```python
from build123d import *

# Parameters (mm, degrees)
SKETCH_1_W      = 48
SKETCH_1_H      = 48
EXTRUDE_1_DEPTH = 60


with BuildPart() as part:
    # 草图1 → 凸台-拉伸1 (new body)
    with BuildSketch(Plane(origin=(0, 0, 0), x_dir=(1, 0, 0), z_dir=(0, 1, 0))):
        Rectangle(SKETCH_1_W, SKETCH_1_H)
    extrude(amount=EXTRUDE_1_DEPTH)

    # Surface Cut 1
    split(bisect_by=Plane(origin=(-14.481029553, 8.36062631, -7.699699993), x_dir=(0.3622245100921348, -0.20913041840877658, -0.9083269633698446), z_dir=(0.7866342252206607, -0.45416348168492593, 0.41826083681754983)), keep=Keep.TOP)


solid = part.part
```
The listing builds one solid part. Answer for the finished solid, in the listing's coordinates (mm). Coordinates: 2 decimals unless noted, no trailing zeros. Loops run counter-clockwise (first coordinate to the right, second up) from the corner with the lowest first, then second, coordinate; pieces in that order, holes last. Notation, with made-up numbers: (41.5, -30.75) - (76.5, -30.75) arc R20 ccw to (76.5, -19.75) - close; hole circle Ø8 at (19.5, 33). An arc over 180 degrees is marked (long way). Use a Markdown table: item, result. Add a question column.
1) The part is cut by section D-D, the plane z = -3. Give the vertices of the cut face in (x, y).
2) The part is cut by section B-B, the plane x = 11.5. Give the vertices of the cut face in (y, z), and give its area (3 significant figures).
3) The part is cut by section C-C, the plane y = 27. Give the vertices of the cut face in (x, z), and give its area (3 significant figures).
4) Find the intervals of material crossed by line 1 (Y direction, x = -6.5, z = 18); line 2 (X direction, y = 49.5, z = 1.5); line 3 (Z direction, x = 6, y = 48.5), in increasing order.
5) The part is cut by section A-A, the plane z = 3. Give the vertices of the cut face in (x, y).
6) Given pin 1 (12 mm diameter, centred on y = 52, z = 9.5, fed in from -X); pin 2 (12 mm diameter, centred on y = 36, z = -7.5, fed in from -X); pin 3 (6 mm diameter, centred on x = -8, z = -17.5, fed in from +Y), each flat-ended and moving along its own axis, determine where each tip first touches the part or whether it passes through.
Here are the results:
| question | item | result |
|---|---|---|
| 1 | outline | (-21.81, 0) - (24, 0) - (24, 60) - (12.83, 60) - close |
| 2 | outline | (0, -24) - (38.35, -24) - (60, -0.49) - (60, 24) - (0, 24) - close |
| 2 | area | 2,630 mm^2 |
| 3 | outline | (-20.57, 24) - (4.95, -24) - (24, -24) - (24, 24) - close |
| 3 | area | 1,530 mm^2 |
| 4 | line 1 | y = 0 to 45.85 |
| 4 | line 2 | x = 4.38 to 24 |
| 4 | line 3 | z = -2.63 to 24 |
| 5 | outline | (-24, 0) - (24, 0) - (24, 60) - (9.64, 60) - (-24, 1.73) - close |
| 6 | pin 1 | stops at x = -3.14 |
| 6 | pin 2 | stops at x = -3.34 |
| 6 | pin 3 | stops at y = 16.45 |
